Here's how the part is built. I have some questions about the finished solid (model axes, mm). Face numbers are marked on the shaded views. Round coordinates to 2 decimals unless told otherwise and drop trailing zeros. Order: outer loops, then holes, each group sorted by start corner. A loop starts at its lowest first (then second) coordinate and runs counter-clockwise, first axis right, second up. Notation, with made-up numbers: (36, 44) - (75, 44) arc R23 cw to (75, 59) - close; hole circle Ø11 at (4, 41.5). An arc over 180 degrees is marked (long way). One line per item, written item: value.
from build123d import *

# Parameters (mm, degrees)
BASENUTSKE_R       = 10
BASENUT_DEPTH      = 10
SKETCH6_OUTSIDE_W  = 84.128
SKETCH6_OUTSIDE_H  = 79.486
SKETCH6_OUTSIDE_R  = 14.25
CUT_EXTRUDE2_DEPTH = 11
CUT_EXTRUDE2_TAPER = 60


with BuildPart() as part:
    # BaseNutSke → BaseNut (new body)
    with BuildSketch(Plane.XY):
        Polygon((8.660254038, -15), (-8.660254038, -15), (-17.320508076, 0), (-8.660254038, 15), (8.660254038, 15), (17.320508076, 0), align=None)
        Circle(BASENUTSKE_R, mode=Mode.SUBTRACT)
    extrude(amount=-BASENUT_DEPTH)

    # Sketch6 outside → Cut-Extrude2 (cut, through all)
    with BuildSketch(Plane(origin=(0, 0, -10), x_dir=(-1, 0, 0), z_dir=(0, 0, -1))):
        Rectangle(SKETCH6_OUTSIDE_W, SKETCH6_OUTSIDE_H)
        Circle(SKETCH6_OUTSIDE_R, mode=Mode.SUBTRACT)
    cut_extrude2 = extrude(amount=-CUT_EXTRUDE2_DEPTH, taper=CUT_EXTRUDE2_TAPER, mode=Mode.SUBTRACT)

    # Mirror1: Cut-Extrude2 across plane
    add(cut_extrude2.mirror(Plane(origin=(0, 0, -5), x_dir=(1, 0, 0), z_dir=(0, 0, -1))), mode=Mode.SUBTRACT)


solid = part.part
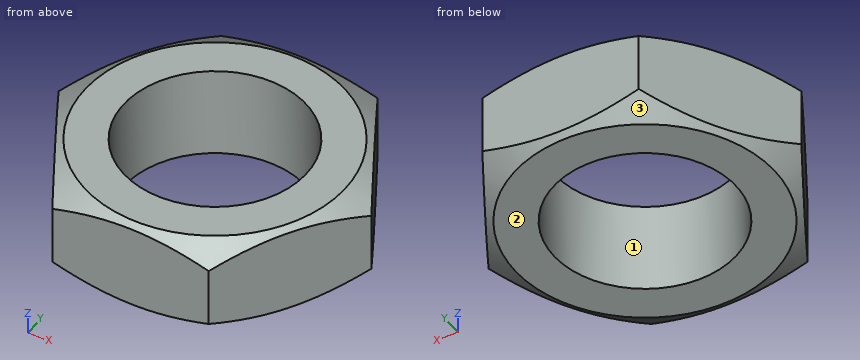
Q1. If I drill on line 1 along Y through (x, z) = (0, -7.25); line 2 along Y through (x, z) = (-5, -3.25); line 3 along X through (y, z) = (0.5, -1.25), over which ranges is the centre line in solid material (lowest first)?
Results list:
line 1: -15 to -10, 10 to 15
line 2: -15 to -8.66, 8.66 to 15
line 3: -16.41 to -9.99, 9.99 to 16.41
Q2. If we section it at A-A, the plane x = 0: Please give me the cut outline in (y, z).
Results list:
outline: (-15, -9.57) - (-14.25, -10) - (-10, -10) - (-10, 0) - (-14.25, 0) - (-15, -0.43) - close; (10, -10) - (14.25, -10) - (15, -9.57) - (15, -0.43) - (14.25, 0) - (10, 0) - close
Q3. We'd pull the mould along Y, two halves only. Please class the marked faces 1, 2 and 3: released by +Y, released by -Y, zero draft, split by the parting line, or undercut.
Results list:
face 1: undercut
face 2: zero draft
face 3: split by the parting line
Q4. Will these pins go through, and if not, where does the flat tip stop? pin 1 (8 mm diameter, centred on x = -6, y = -1.5, fed in from -Z); pin 2 (2 mm diameter, centred on x = -12.5, z = -8.5, fed in from +Y); pin 3 (5 mm diameter, centred on y = -8.5, z = -1, fed in from +X); pin 4 (2 mm diameter, centred on x = -11.5, z = -4, fed in from -Y).
Results list:
pin 1: z = -10
pin 2: y = 10.08
pin 3: x = 13.86
pin 4: y = -11.81
